Here's how the part is built. I have some questions about the finished solid (model axes, mm). Face numbers are marked on the shaded views. A direction names the side the tool comes from. Give positions to 0.01 mm unless a question says otherwise; leave off trailing zeros. Loops run counter-clockwise (first coordinate to the right, second up) from the corner with the lowest first, then second, coordinate; pieces in that order, holes last. Notation, with made-up numbers: (-12.5, -20.5) - (7.5, -20.5) arc R6 cw to (7.5, -16.5) - close; hole circle Ø11 at (34, 15). An arc over 180 degrees is marked (long way). Use one line per item in the form item = value.
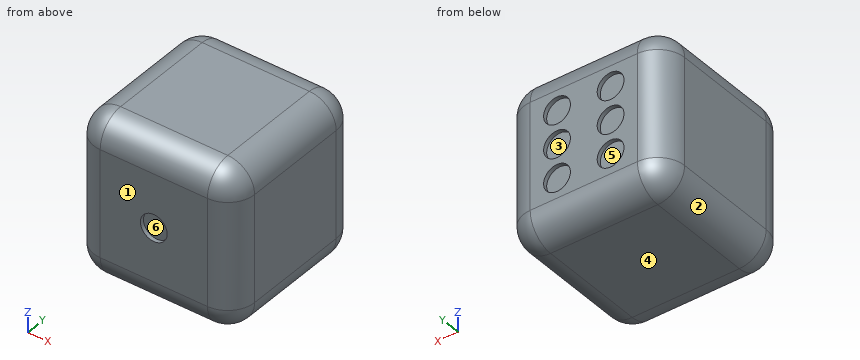
from build123d import *

# Parameters (mm, degrees)
F0_W          = 12
F0_H          = 12
F1_DEPTH      = 6
F1_DEPTH_BACK = 6
F2_R          = 2
F3_R          = 1
F4_DEPTH      = 0.3
F5_R          = 1
F6_DEPTH      = 0.3


with BuildPart() as f1:
    # F0 (on Front) → F1 (new body, two sides)
    with BuildSketch(Plane.XZ) as f1_sk:
        Rectangle(F0_W, F0_H)
    extrude(amount=F1_DEPTH)
    extrude(f1_sk.sketch, amount=-F1_DEPTH_BACK)

    # F2
    f2_edges = [f1.edges().sort_by_distance(p)[0] for p in [
        (6, 0, -6),
        (0, 6, 6),
        (-6, 6, 0),
        (0, 6, -6),
        (6, 6, 0),
        (6, 0, 6),
        (-6, 0, 6),
        (0, -6, -6),
        (-6, 0, -6),
        (-6, -6, 0),
        (0, -6, 6),
        (6, -6, 0),
    ]]
    fillet(f2_edges, radius=F2_R)

    # F3 (on face) → F4 (cut)
    with BuildSketch(Plane.XZ.offset(6)):
        Circle(F3_R)
    extrude(amount=-F4_DEPTH, mode=Mode.SUBTRACT)

    # F5 (on face) → F6 (cut)
    with BuildSketch(Plane(origin=(0, 6, 0), x_dir=(-1, 0, 0), z_dir=(0, 1, 0))):
        with Locations((-2, 2.5)):
            Circle(F5_R)
        with Locations((2, 2.5)):
            Circle(F5_R)
        with Locations((2, 0)):
            Circle(F5_R)
        with Locations((2, -2.5)):
            Circle(F5_R)
        with Locations((-2, 0)):
            Circle(F5_R)
        with Locations((-2, -2.5)):
            Circle(F5_R)
    extrude(amount=-F6_DEPTH, mode=Mode.SUBTRACT)


solid = f1.part
(1) For the marked faces 4, 5 and 6, which set-ups out of +Z, -Z, +X, -X, +Y, -Y let a thin tool reach every point of the face, with its end or its side?
Geometry says:
face_4 = -Z, +X, -X, +Y, -Y
face_5 = +Y
face_6 = -Y
(2) If we section it at C-C (y = 0.5): List the corners of the cut face in (x, z) for me.
Geometry says:
outline = (-6, -4) arc R2 ccw to (-4, -6) - (4, -6) arc R2 ccw to (6, -4) - (6, 4) arc R2 ccw to (4, 6) - (-4, 6) arc R2 ccw to (-6, 4) - close
(3) If we section it at D-D (x = 2): List the corners of the cut face in (y, z) for me.
Geometry says:
outline = (-6, -4) arc R2 ccw to (-4, -6) - (4, -6) arc R2 ccw to (6, -4) - (6, -3.5) - (5.7, -3.5) - (5.7, -1.5) - (6, -1.5) - (6, -1) - (5.7, -1) - (5.7, 1) - (6, 1) - (6, 1.5) - (5.7, 1.5) - (5.7, 3.5) - (6, 3.5) - (6, 4) arc R2 ccw to (4, 6) - (-4, 6) arc R2 ccw to (-6, 4) - close
(4) For P1, Ø0.6, axis at x = 2, z = 2, coming from the +Y side; P2, Ø1.2, axis at x = 0, z = 0, coming from the -Y side, each with a flat end and sliding along its axis, tell me the tip position at first contact or that it passes through.
Geometry says:
P1 = 5.7
P2 = -5.7
(5) If I drill on probe 1 along Y at (x, z) = (-2, -2); probe 2 along Z at (x, y) = (2, 5.8); probe 3 along Y at (x, z) = (-1, 4.5), over which ranges is the centre line in solid material (lowest first)?
Geometry says:
probe_1 = -6 to 5.7
probe_2 = -4.87 to -3.5, -1.5 to -1, 1 to 1.5, 3.5 to 4.87
probe_3 = -5.94 to 5.94
(6) Thinking about a two-plate mould opening in X: for the marked faces 1, 2 and 3, which applies, pulls with the +X half, pulls with the -X half, needs draft (parallel to the pull), parting line crosses it, or undercut?
Geometry says:
face_1 = needs draft
face_2 = pulls with the -X half
face_3 = undercut
